Here's how the part is built. I have some questions about the finished solid (model axes, mm). Face numbers are marked on the shaded views. A direction names the side the tool comes from. Give positions to 0.01 mm unless a question says otherwise; leave off trailing zeros. Write each loop counter-clockwise with the first axis right and the second up, starting at its lowest first coordinate (ties: lowest second). Pieces come first, ordered by that corner, then holes. Notation, with made-up numbers: (57, -10.5) -> (114, -10.5) arc R8 ccw to (114, -1.5) -> close; hole circle Ø2 at (82.5, 31). An arc over 180 degrees is marked (long way). Put each result on its own line as item: value. Start each with the question number.
from build123d import *

# Parameters (mm, degrees)
F0_W      = 127
F0_H      = 25.4
F1_DEPTH  = 25.4
F2_DEPTH  = 126.8292367458
F3_W      = 88.223606348
F3_H      = 12.3776346445
F4_DEPTH  = 152.2302367458
F5_R      = 2.38125
F6_DEPTH  = 127.001
F7_R      = 2.38125
F8_DEPTH  = 127.001
F9_W      = 45.556999743
F9_H      = 18.5132399201
F9_W_2    = 45.3319624066
F9_H_2    = 16.7129561305
F9_W_3    = 15.3134018183
F9_H_3    = 63.6049769819
F10_DEPTH = 13.0233653555


with BuildPart() as f1:
    # F0 (on Right) → F1 (new body)
    with BuildSketch(Plane.YZ):
        with Locations((-63.5, 12.7)):
            Rectangle(F0_W, F0_H)
    extrude(amount=F1_DEPTH)

    # F2 (add): a face of the model
    f2_faces = [f1.faces().sort_by_distance(p)[0] for p in [
        (25.4, -63.5, 12.7),
    ]]
    extrude(f2_faces, amount=F2_DEPTH)

    # F3 (on face) → F4 (cut, through all)
    with BuildSketch(Plane.YZ.offset(152.2292367458)):
        with Locations((-61.8745535612, 6.1888173223)):
            Rectangle(F3_W, F3_H)
    extrude(amount=-F4_DEPTH, mode=Mode.SUBTRACT)

    # F5 (on face) → F6 (cut, through all)
    with BuildSketch(Plane.XZ.offset(127)):
        with Locations((147.4088132381, 3.7022531033)):
            Circle(F5_R)
    extrude(amount=-F6_DEPTH, mode=Mode.SUBTRACT)

    # F7 (on face) → F8 (cut, through all)
    with BuildSketch(Plane.XZ.offset(127)):
        with Locations((5.9837484732, 4.8569738865)):
            Circle(F7_R)
    extrude(amount=-F8_DEPTH, mode=Mode.SUBTRACT)

    # F9 (on face) → F10 (cut, through all)
    with BuildSketch(Plane(origin=(0, 0, 12.3776346445), x_dir=(1, 0, 0), z_dir=(0, 0, -1))):
        with Locations((22.7784998715, 86.0507525504)):
            Rectangle(F9_W, F9_H)
        with Locations((22.6659812033, 45.3535504639)):
            Rectangle(F9_W_2, F9_H_2)
        with Locations((122.6406171918, 62.9230011255)):
            Rectangle(F9_W_3, F9_H_3)
    extrude(amount=-F10_DEPTH, mode=Mode.SUBTRACT)


solid = f1.part
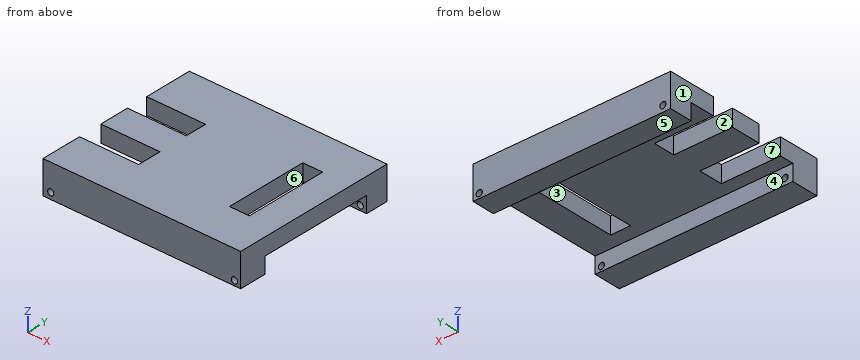
1) I want a section at A-A, the plane y = -92.5. Write out the boundary of the cut face in (x, z).
2) I want a section at B-B, the plane x = 25.5. Write out the boundary of the cut face in (y, z).
3) I'm going to push flat-ended pins straight in: pin 1 Ø6.5 at (y, z) = (-83, 19) entering from -X; pin 2 Ø3 at (x, y) = (55.5, -60) entering from -Z; pin 3 Ø10.5 at (y, z) = (-43.5, 20.5) entering from -X. Where does each tip first touch, or does it pass through?
4) Which directions (+Z, -Z, +X, -X, +Y, -Y) give clear straight access to the entire face, cutting with the end or side of a thin tool? Please do the marked faces 4, 5, 6 and 7.
5) I need wall thicknesses on probe 1 along Y at (x, z) = (25, 14); probe 2 along X at (y, z) = (-48.5, 20.25); probe 3 along Y at (x, z) = (85.5, 2.75). Which ranges of each line are inside material? Lowest first, please.
6) I want a section at D-D, the plane z = 21.25. Write out the boundary of the cut face in (x, y), and give its area (3 significant figures).
7) Thinking about a two-plate mould opening in X: for the marked faces 1, 2 and 3, which applies, released by +X, released by -X, zero draft, split by the parting line, or undercut?
8) I want a section at C-C, the plane x = 122. Write out the boundary of the cut face in (y, z).
Established:
1. outline: (45.56, 12.38) -> (114.98, 12.38) -> (114.98, 25.4) -> (45.56, 25.4) -> close; (130.3, 12.38) -> (152.23, 12.38) -> (152.23, 25.4) -> (130.3, 25.4) -> close
2. outline: (-127, 0) -> (-105.99, 0) -> (-105.99, 12.38) -> (-95.31, 12.38) -> (-95.31, 25.4) -> (-127, 25.4) -> close; (-76.79, 12.38) -> (-53.71, 12.38) -> (-53.71, 25.4) -> (-76.79, 25.4) -> close; (-37, 12.38) -> (-17.76, 12.38) -> (-17.76, 0) -> (0, 0) -> (0, 25.4) -> (-37, 25.4) -> close
3. pin 1: stops at x = 45.56
3. pin 2: stops at z = 12.38
3. pin 3: stops at x = 45.33
4. face 4: -Z, +X, -X
4. face 5: -Z, +X, -X, +Y, -Y
4. face 6: +Z, -Z
4. face 7: +Z, -Z, -X
5. probe 1: y = -127 to -95.31, -76.79 to -53.71, -37 to 0
5. probe 2: x = 45.33 to 114.98, 130.3 to 152.23
5. probe 3: y = -127 to -105.99, -17.76 to 0
6. outline: (0, -127) -> (152.23, -127) -> (152.23, 0) -> (0, 0) -> (0, -37) -> (45.33, -37) -> (45.33, -53.71) -> (0, -53.71) -> (0, -76.79) -> (45.56, -76.79) -> (45.56, -95.31) -> (0, -95.31) -> close; hole (114.98, -94.73) -> (130.3, -94.73) -> (130.3, -31.12) -> (114.98, -31.12) -> close
6. area: 16,800 mm2
7. face 1: released by -X
7. face 2: zero draft
7. face 3: undercut
8. outline: (-127, 0) -> (-105.99, 0) -> (-105.99, 12.38) -> (-94.73, 12.38) -> (-94.73, 25.4) -> (-127, 25.4) -> close; (-31.12, 12.38) -> (-17.76, 12.38) -> (-17.76, 0) -> (0, 0) -> (0, 25.4) -> (-31.12, 25.4) -> close
